Can you work these out from the model? Positions are in its coordinate system, mm. A direction names the side the tool comes from. Round coordinates to 2 decimals unless told otherwise and drop trailing zeros. Return JSON: item names as keys, results as strings.
```python
from build123d import *

# Parameters (mm, degrees)
BOSS_EXTRUDE1_DEPTH                             = 9.6
CSK_FOR_M3_FLAT_HEAD_MACHINE_SCREW1_D           = 3.4
CSK_FOR_M3_FLAT_HEAD_MACHINE_SCREW1_CSINK_D     = 6.3
CSK_FOR_M3_FLAT_HEAD_MACHINE_SCREW1_CSINK_ANGLE = 90
M3X0_5_TAPPED_HOLE1_D                           = 2.5
M3X0_5_TAPPED_HOLE1_DEPTH                       = 6.748924226
M3X0_5_TAPPED_HOLE1_TIP                         = 0.751075774


with BuildPart() as part:
    # Sketch2 → Boss-Extrude1 (new body)
    with BuildSketch(Plane(origin=(0, 0, 0), x_dir=(0, 0, -1), z_dir=(1, 0, 0))):
        with BuildLine():
            Line((-34.1, -38.1), (34.1, -38.1))
            ThreePointArc((34.1, -38.1), (36.928427125, -36.928427125), (38.1, -34.1))
            Line((38.1, -34.1), (38.1, 34.1))
            ThreePointArc((38.1, 34.1), (36.928427125, 36.928427125), (34.1, 38.1))
            Line((34.1, 38.1), (-34.1, 38.1))
            ThreePointArc((-34.1, 38.1), (-36.928427125, 36.928427125), (-38.1, 34.1))
            Line((-38.1, 34.1), (-38.1, -34.1))
            ThreePointArc((-38.1, -34.1), (-36.928427125, -36.928427125), (-34.1, -38.1))
        make_face()
    extrude(amount=BOSS_EXTRUDE1_DEPTH)

    # CSK for M3 Flat Head Machine Screw1 (through all)
    with Locations(Plane(origin=(9.6, 0, 0), x_dir=(0, 0, 1), z_dir=(1, 0, 0))):
        with Locations((-34.100008, -34.1), (34.1, -34.1), (34.1, 34.1), (-34.100008, 34.1), (0, -34.94999995), (34.95, 0), (0, 34.95), (-34.95, 0)):
            CounterSinkHole(CSK_FOR_M3_FLAT_HEAD_MACHINE_SCREW1_D / 2, CSK_FOR_M3_FLAT_HEAD_MACHINE_SCREW1_CSINK_D / 2, counter_sink_angle=CSK_FOR_M3_FLAT_HEAD_MACHINE_SCREW1_CSINK_ANGLE)

    # M3x0.5 Tapped Hole1
    with Locations(Plane(origin=(9.6, 0, 0), x_dir=(0, 0, -1), z_dir=(1, 0, 0))):
        with Locations((-25, 25), (25, 25), (25, -25), (-25, -25)):
            Hole(M3X0_5_TAPPED_HOLE1_D / 2, depth=M3X0_5_TAPPED_HOLE1_DEPTH)
            with Locations((0, 0, -(M3X0_5_TAPPED_HOLE1_DEPTH + M3X0_5_TAPPED_HOLE1_TIP / 2))):  # 118° drill point
                Cone(0, M3X0_5_TAPPED_HOLE1_D / 2, M3X0_5_TAPPED_HOLE1_TIP, mode=Mode.SUBTRACT)


solid = part.part
```
Q1. Suppose I cut it at A-A, the plane x = 4.75. State how many separate pieces and enclosed holes the cut face has, plus the area to 3 significant figures.
Results:
{"separate pieces": "1", "enclosed holes": "12", "area": "5,700 mm2"}
Q2. On a 3-axis mill with a long thin cutter (end or side, diameter ignored), from which of +Z, -Z, +X, -X, +Y, -Y can I reach the whole of each face in a straight line? I mean faces 1 (the flat face through (5, 0, 38.1)), 2 (the cylindrical face through (6.178, -25.479, 26.155)). Say none if no direction works.
Results:
{"face 1": "+Z, +X, -X, +Y, -Y", "face 2": "+X"}
Q3. I'm going to push a flat-ended pin straight in: pin 1 Ø4 at (y, z) = (0, 34.95) entering from +X. Where does the tip first touch, or does it pass through?
Results:
{"pin 1": "stops at x = 8.45"}
Q4. If I drill on line 1 along Y through (x, z) = (4.5, -25); line 2 along Y through (x, z) = (4.5, 34.1), over which ranges is the centre line in solid material (lowest first)?
Results:
{"line 1": "y = -38.1 to -26.25, -23.75 to 23.75, 26.25 to 38.1", "line 2": "y = -38.1 to -35.8, -32.4 to -1.47, 1.47 to 32.4, 35.8 to 38.1"}
